from build123d import *

# Parameters (mm, degrees)
F0_R         = 6.35
F1_DEPTH     = 12.7
F2_T2_ANGLE  = 99.446116479
F2_T4_ANGLE  = 59.2916827944
F2_T6_ANGLE  = 201.7148311049
F2_T8_ANGLE  = 200.3212768017
F2_T10_ANGLE = 94.2324188496
F2_T12_ANGLE = 210.9341102164
F2_T14_ANGLE = 94.2324188496
F2_T16_ANGLE = 210.9341102164
F2_T18_ANGLE = 200.3212768017
F2_T20_ANGLE = 59.2916827944
F2_T22_ANGLE = 201.7148311049
F2_T24_ANGLE = 99.446116479


# Not quite as in the source:
# - a fillet or chamfer that OpenCascade refuses, or shapes differently, is made with other operations: its cross-section is extruded or revolved along the edge and cut away or added


with BuildPart() as f1:
    # F0 (on Top) → F1 (new body)
    with BuildSketch(Plane.XY):
        with BuildLine():
            ThreePointArc((-23.0979636954, -28.8973481426), (-12.2116587197, -18.0861984821), (2.0883176929, -12.527127732))
            ThreePointArc((2.0883176929, -12.527127732), (-10.0506029407, -7.7637220795), (-11.5934607492, 5.1847534038))
            ThreePointArc((-11.5934607492, 5.1847534038), (-20.2173700121, -8.8847131705), (-32.1537121721, -20.2796873478))
            ThreePointArc((-32.1537121721, -20.2796873478), (-25.5280345903, -19.7355993147), (-22.0480633142, -25.4))
            ThreePointArc((-22.0480633142, -25.4), (-22.3161995958, -27.2257693475), (-23.0979636954, -28.8973481426))
        make_face()
        with BuildLine():
            ThreePointArc((10.5830984733, 7.0205431916), (12.1592629425, 3.6663775985), (12.7, 0))
            ThreePointArc((12.7, 0), (9.6905013983, -8.2087869171), (2.0883176929, -12.527127732))
            ThreePointArc((2.0883176929, -12.527127732), (17.4183090092, -13.1467749254), (31.2229657331, -19.8418514101))
            ThreePointArc((31.2229657331, -19.8418514101), (29.2220209534, -12.4165925694), (35.8447458338, -8.5079145294))
            ThreePointArc((35.8447458338, -8.5079145294), (21.5024747262, -3.5278630909), (10.5830984733, 7.0205431916))
        make_face()
        with BuildLine():
            ThreePointArc((-11.5934607492, 5.1847534038), (-1.0477304131, 12.6567081416), (10.5830984733, 7.0205431916))
            ThreePointArc((10.5830984733, 7.0205431916), (5.1104904876, 21.1821889646), (6.0989820006, 36.3322560831))
            ThreePointArc((6.0989820006, 36.3322560831), (-0.5872613397, 31.7772138958), (-6.320221624, 37.4857536138))
            ThreePointArc((-6.320221624, 37.4857536138), (-6.8559724512, 20.992280129), (-11.5934607492, 5.1847534038))
        make_face()
        with BuildLine():
            ThreePointArc((2.0883176929, -12.527127732), (9.6905013983, -8.2087869171), (12.7, 0))
            ThreePointArc((12.7, 0), (12.1592629425, 3.6663775985), (10.5830984733, 7.0205431916))
            ThreePointArc((10.5830984733, 7.0205431916), (-1.0477304131, 12.6567081416), (-11.5934607492, 5.1847534038))
            ThreePointArc((-11.5934607492, 5.1847534038), (-10.0506029407, -7.7637220795), (2.0883176929, -12.527127732))
        make_face()
        Circle(F0_R, mode=Mode.SUBTRACT)
        with BuildLine():
            ThreePointArc((-32.1537121721, -20.2796873478), (-32.7755456308, -30.0000161487), (-23.0979636954, -28.8973481426))
            ThreePointArc((-23.0979636954, -28.8973481426), (-22.3161995958, -27.2257693475), (-22.0480633142, -25.4))
            ThreePointArc((-22.0480633142, -25.4), (-25.5280345903, -19.7355993147), (-32.1537121721, -20.2796873478))
        make_face()
        with BuildLine():
            ThreePointArc((41.4519366858, -14.8143187798), (39.8474260225, -10.5949786709), (35.8447458338, -8.5079145294))
            ThreePointArc((35.8447458338, -8.5079145294), (29.2220209534, -12.4165925694), (31.2229657331, -19.8418514101))
            ThreePointArc((31.2229657331, -19.8418514101), (37.9029217313, -20.5131768035), (41.4519366858, -14.8143187798))
        make_face()
        with BuildLine():
            ThreePointArc((-6.320221624, 37.4857536138), (-0.5872613397, 31.7772138958), (6.0989820006, 36.3322560831))
            ThreePointArc((6.0989820006, 36.3322560831), (6.2869323085, 37.2072614336), (6.35, 38.1))
            ThreePointArc((6.35, 38.1), (-0.3074838917, 44.442551037), (-6.320221624, 37.4857536138))
        make_face()
    extrude(amount=F1_DEPTH)

    # F2: fillet of radius 5.08 on 12 edges, made by hand

    # F2_s1 → F2_t2 (revolve, cut)
    with BuildSketch(Plane(origin=(36.3426576492, -4.2806736606, 0), x_dir=(0, 0, 1), z_dir=(0.9931345276, -0.1169778186, 0))):
        with BuildLine():
            ThreePointArc((7.62, 4.2564635014), (11.2121024484, 5.744361053), (12.7, 9.3364635014))
            Line((12.7, 9.3364635014), (12.7, 4.2564635014))
            Line((12.7, 4.2564635014), (7.62, 4.2564635014))
        make_face()
    revolve(axis=Axis((39.9699722036, 26.5150051248, 12.7), (0, 0, -1)), revolution_arc=F2_T2_ANGLE, mode=Mode.SUBTRACT)

    # F2_s3 → F2_t4 (revolve, cut)
    with BuildSketch(Plane(origin=(-3.6681952371, 37.7434973641, 0), x_dir=(0, 0, 1), z_dir=(-0.0967317144, 0.995310492, 0))):
        with BuildLine():
            ThreePointArc((7.62, -2.6645216828), (11.2121024484, -1.1766241312), (12.7, 2.4154783172))
            Line((12.7, 2.4154783172), (12.7, -2.6645216828))
            Line((12.7, -2.6645216828), (7.62, -2.6645216828))
        make_face()
    revolve(axis=Axis((-69.9851672009, 31.2983182556, 12.7), (0, 0, -1)), revolution_arc=F2_T4_ANGLE, mode=Mode.SUBTRACT)

    # F2_s5 → F2_t6 (revolve, cut)
    with BuildSketch(Plane(origin=(10.1871858245, 35.1473210497, 0), x_dir=(0, 0, 1), z_dir=(-0.2783848688, -0.9604696064, 0))):
        with BuildLine():
            ThreePointArc((7.62, 4.2564635014), (11.2121024484, 5.744361053), (12.7, 9.3364635014))
            Line((12.7, 9.3364635014), (12.7, 4.2564635014))
            Line((12.7, 4.2564635014), (7.62, 4.2564635014))
        make_face()
    revolve(axis=Axis((0, 38.1, 12.7), (0, 0, 1)), revolution_arc=F2_T6_ANGLE, mode=Mode.SUBTRACT)

    # F2_s7 → F2_t8 (revolve, cut)
    with BuildSketch(Plane(origin=(-30.5778054296, -22.4282202745, 0), x_dir=(0, 0, 1), z_dir=(0.8063484492, 0.591440765, 0))):
        with BuildLine():
            ThreePointArc((7.62, -2.6645216828), (11.2121024484, -1.1766241312), (12.7, 2.4154783172))
            Line((12.7, 2.4154783172), (12.7, -2.6645216828))
            Line((12.7, -2.6645216828), (7.62, -2.6645216828))
        make_face()
    revolve(axis=Axis((-28.3980633142, -25.4, 12.7), (0, 0, 1)), revolution_arc=F2_T8_ANGLE, mode=Mode.SUBTRACT)

    # F2_s9 → F2_t10 (revolve, cut)
    with BuildSketch(Plane(origin=(-20.2906858047, -30.7497714597, 0), x_dir=(0, 0, 1), z_dir=(-0.550763487, -0.8346613573, 0))):
        with BuildLine():
            ThreePointArc((5.08, 3.3633735001), (1.4878975516, 4.8512710517), (0, 8.4433735001))
            Line((0, 8.4433735001), (0, 3.3633735001))
            Line((0, 3.3633735001), (5.08, 3.3633735001))
        make_face()
    revolve(axis=Axis((8.2675580223, -49.5943457482, 0), (0, 0, -1)), revolution_arc=F2_T10_ANGLE, mode=Mode.SUBTRACT)

    # F2_s11 → F2_t12 (revolve, cut)
    with BuildSketch(Plane(origin=(29.1684101252, -22.5047600746, 0), x_dir=(0, 0, 1), z_dir=(-0.7917374221, 0.6108615673, 0))):
        with BuildLine():
            ThreePointArc((5.08, 3.3633735001), (1.4878975516, 4.8512710517), (0, 8.4433735001))
            Line((0, 8.4433735001), (0, 3.3633735001))
            Line((0, 3.3633735001), (5.08, 3.3633735001))
        make_face()
    revolve(axis=Axis((35.1019366858, -14.8143187798, 0), (0, 0, 1)), revolution_arc=F2_T12_ANGLE, mode=Mode.SUBTRACT)

    # F2_s13 → F2_t14 (revolve, cut)
    with BuildSketch(Plane(origin=(-20.2906858047, -30.7497714597, 0), x_dir=(0, 0, 1), z_dir=(-0.550763487, -0.8346613573, 0))):
        with BuildLine():
            ThreePointArc((7.62, 3.3633735001), (11.2121024484, 4.8512710517), (12.7, 8.4433735001))
            Line((12.7, 8.4433735001), (12.7, 3.3633735001))
            Line((12.7, 3.3633735001), (7.62, 3.3633735001))
        make_face()
    revolve(axis=Axis((8.2675580223, -49.5943457482, 12.7), (0, 0, -1)), revolution_arc=F2_T14_ANGLE, mode=Mode.SUBTRACT)

    # F2_s15 → F2_t16 (revolve, cut)
    with BuildSketch(Plane(origin=(29.1684101252, -22.5047600746, 0), x_dir=(0, 0, 1), z_dir=(-0.7917374221, 0.6108615673, 0))):
        with BuildLine():
            ThreePointArc((7.62, 3.3633735001), (11.2121024484, 4.8512710517), (12.7, 8.4433735001))
            Line((12.7, 8.4433735001), (12.7, 3.3633735001))
            Line((12.7, 3.3633735001), (7.62, 3.3633735001))
        make_face()
    revolve(axis=Axis((35.1019366858, -14.8143187798, 12.7), (0, 0, 1)), revolution_arc=F2_T16_ANGLE, mode=Mode.SUBTRACT)

    # F2_s17 → F2_t18 (revolve, cut)
    with BuildSketch(Plane(origin=(-30.5778054296, -22.4282202745, 0), x_dir=(0, 0, 1), z_dir=(0.8063484492, 0.591440765, 0))):
        with BuildLine():
            ThreePointArc((5.08, -2.6645216828), (1.4878975516, -1.1766241312), (0, 2.4154783172))
            Line((0, 2.4154783172), (0, -2.6645216828))
            Line((0, -2.6645216828), (5.08, -2.6645216828))
        make_face()
    revolve(axis=Axis((-28.3980633142, -25.4, 0), (0, 0, 1)), revolution_arc=F2_T18_ANGLE, mode=Mode.SUBTRACT)

    # F2_s19 → F2_t20 (revolve, cut)
    with BuildSketch(Plane(origin=(-3.6681952371, 37.7434973641, 0), x_dir=(0, 0, 1), z_dir=(-0.0967317144, 0.995310492, 0))):
        with BuildLine():
            ThreePointArc((5.08, -2.6645216828), (1.4878975516, -1.1766241312), (0, 2.4154783172))
            Line((0, 2.4154783172), (0, -2.6645216828))
            Line((0, -2.6645216828), (5.08, -2.6645216828))
        make_face()
    revolve(axis=Axis((-69.9851672009, 31.2983182556, 0), (0, 0, -1)), revolution_arc=F2_T20_ANGLE, mode=Mode.SUBTRACT)

    # F2_s21 → F2_t22 (revolve, cut)
    with BuildSketch(Plane(origin=(10.1871858245, 35.1473210497, 0), x_dir=(0, 0, 1), z_dir=(-0.2783848688, -0.9604696064, 0))):
        with BuildLine():
            ThreePointArc((5.08, 4.2564635014), (1.4878975516, 5.744361053), (0, 9.3364635014))
            Line((0, 9.3364635014), (0, 4.2564635014))
            Line((0, 4.2564635014), (5.08, 4.2564635014))
        make_face()
    revolve(axis=Axis((0, 38.1, 0), (0, 0, 1)), revolution_arc=F2_T22_ANGLE, mode=Mode.SUBTRACT)

    # F2_s23 → F2_t24 (revolve, cut)
    with BuildSketch(Plane(origin=(36.3426576492, -4.2806736606, 0), x_dir=(0, 0, 1), z_dir=(0.9931345276, -0.1169778186, 0))):
        with BuildLine():
            ThreePointArc((5.08, 4.2564635014), (1.4878975516, 5.744361053), (0, 9.3364635014))
            Line((0, 9.3364635014), (0, 4.2564635014))
            Line((0, 4.2564635014), (5.08, 4.2564635014))
        make_face()
    revolve(axis=Axis((39.9699722036, 26.5150051248, 0), (0, 0, -1)), revolution_arc=F2_T24_ANGLE, mode=Mode.SUBTRACT)


solid = f1.part
Part model, mm, in its own coordinate system. Coordinates: 2 decimals unless noted, no trailing zeros. Order: outer loops, then holes, each group sorted by start corner. A loop starts at its lowest first (then second) coordinate and runs counter-clockwise, first axis right, second up. Notation, with made-up numbers: M 29,59.25 L 66,59.25 A11 cw 66,76.25 Z; hole C 60,11 d9. An arc over 180 degrees is marked long. One line per question, with ' | ' between items.
Q1. Slice it at A-A (z = 6.5). Give the cut face in (x, y) (3 decimals), and give its area (3 significant figures).
A:
outline: M -32.154,-20.28 A6.35 ccw long -23.098,-28.897 A37.579 cw 31.223,-19.842 A6.35 ccw long 35.845,-8.508 A35.265 cw 6.099,36.332 A6.35 ccw long -6.32,37.486 A63.965 cw Z; hole C 0,0 d12.7 | area: 1,540 mm^2
Q2. Pin check, flat tips, straight feed: P1, Ø1.5, axis at x = -16.5, z = 4, coming from the -Y side; P2, Ø6, axis at y = 19.5, z = 2, coming from the +X side; P3, Ø1.5, axis at x = -26, z = 2, coming from the +Y side; P4, Ø5, axis at x = 1.5, y = 2.5, coming from the -Z side. Stop position of each tip, or through.
A:
P1: stops at y = -21.88 | P2: stops at x = 5.82 | P3: stops at y = -15.58 | P4: passes through
Q3. Two-plate mould, pull along Y, no slides. Class faces 1 (the face through (-32.89, -29.89, 6.33)), 2 (the face through (34, -14, 0)), 3 (the face through (-1.38, -6.2, 6.26)): +Y half, -Y half, draft (parallel to the pull), parting line (faces both ways), or undercut.
A:
face 1: parting line | face 2: draft | face 3: undercut
Q4. Drill centre lines: line 1 (Y direction, x = 0, z = 8.25); line 2 (Y direction, x = 0, z = 9.5); line 3 (X direction, y = 13, z = 11.5). Where is each one in solid material? Low to high.
A:
line 1: y = -12.9 to -6.35, 6.35 to 44.41 | line 2: y = -12.57 to -6.35, 6.35 to 44.09 | line 3: x = -6.82 to 5.46
